Read the model definition and answer for the solid it produces. Units are mm, in the model's axes. Face numbers are marked on the shaded views. Coordinates: 2 decimals unless noted, no trailing zeros. Loops run counter-clockwise (first coordinate to the right, second up) from the corner with the lowest first, then second, coordinate; pieces in that order, holes last.
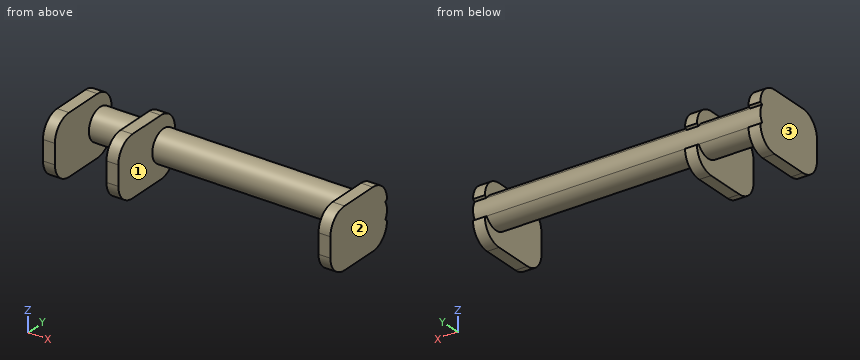
from build123d import *

# Parameters (mm, degrees)
SCHIZZO1_R                   = 8
ESTRUSIONE_ESTRUSIONE1_DEPTH = 145
ESTRUSIONE_ESTRUSIONE2_DEPTH = 6
RIPETIZIONE_A_L1_COUNT       = 2
RIPETIZIONE_A_L1_PITCH       = 32
RIPETIZIONE_A_L2_COUNT       = 2
RIPETIZIONE_A_L2_PITCH       = 139
EXTRUDE2_DEPTH               = 150.244765402


with BuildPart() as part:
    # Schizzo1 → Estrusione-Estrusione1 (new body)
    with BuildSketch(Plane(origin=(0, 0, 0), x_dir=(0, 0, -1), z_dir=(1, 0, 0))):
        Circle(SCHIZZO1_R)
    extrude(amount=ESTRUSIONE_ESTRUSIONE1_DEPTH)

    # Schizzo2 → Estrusione-Estrusione2 (add)
    with BuildSketch(Plane.ZY):
        with BuildLine():
            Line((-5, 8), (5, 8))
            ThreePointArc((5, 8), (12.071067812, 5.071067812), (15, -2))
            Line((15, -2), (15, -22))
            ThreePointArc((15, -22), (12.071067812, -29.071067812), (5, -32))
            Line((5, -32), (-5, -32))
            ThreePointArc((-5, -32), (-12.071067812, -29.071067812), (-15, -22))
            Line((-15, -22), (-15, -2))
            ThreePointArc((-15, -2), (-12.071067812, 5.071067812), (-5, 8))
        make_face()
    estrusione_estrusione2 = extrude(amount=-ESTRUSIONE_ESTRUSIONE2_DEPTH)

    # Ripetizione a L1: Estrusione-Estrusione2 ×2
    with Locations(*[(i * RIPETIZIONE_A_L1_PITCH, 0, 0) for i in range(1, RIPETIZIONE_A_L1_COUNT)]):
        add(estrusione_estrusione2)

    # Ripetizione a L2: Estrusione-Estrusione2 ×2
    with Locations(*[(i * RIPETIZIONE_A_L2_PITCH, 0, 0) for i in range(1, RIPETIZIONE_A_L2_COUNT)]):
        add(estrusione_estrusione2)

    # Sketch1 → Extrude2 (cut, through all)
    with BuildSketch(Plane.ZY):
        with BuildLine():
            Line((-5, 8), (-4.23999152, 6.783986432))
            ThreePointArc((-4.23999152, 6.783986432), (0, 8), (4.23999152, 6.783986432))
            Line((4.23999152, 6.783986432), (5, 8))
            Line((5, 8), (5, 8.502646834))
            Line((5, 8.502646834), (-5, 8.502646834))
            Line((-5, 8.502646834), (-5, 8))
        make_face()
    extrude(amount=-EXTRUDE2_DEPTH, mode=Mode.SUBTRACT)


solid = part.part
Item 1: A cutting plane is placed at C-C on z = 0. Determine the outline of the cut face in (x, y), then the cut area to 3 significant figures.
Numbers:
outline: (0, -32) - (6, -32) - (6, -8) - (32, -8) - (32, -32) - (38, -32) - (38, -8) - (139, -8) - (139, -32) - (145, -32) - (145, 8) - (0, 8) - close
area: 2,750 mm2
Item 2: A cutting plane is placed at B-B on y = -11.5. Determine the outline of the cut face in (x, z), then the cut area to 3 significant figures.
Numbers:
outline: (0, -15) - (6, -15) - (6, 15) - (0, 15) - close; (32, -15) - (38, -15) - (38, 15) - (32, 15) - close; (139, -15) - (145, -15) - (145, 15) - (139, 15) - close
area: 540 mm2
Item 3: Determine the mould class of the marked faces 1, 2 and 3 for opening direction X: released by +X, released by -X, zero draft, split by the parting line, or undercut.
Numbers:
face 1: undercut
face 2: released by +X
face 3: released by -X
Item 4: Given pin 1 (12 mm diameter, centred on x = 20, z = -2, fed in from -Y); pin 2 (12 mm diameter, centred on x = 17.5, y = -4.5, fed in from -Z); pin 3 (9 mm diameter, centred on y = -14, z = -3.5, fed in from -X); pin 4 (4 mm diameter, centred on x = 103.5, z = 6, fed in from +Y), each flat-ended and moving along its own axis, determine where each tip first touches the part or whether it passes through.
Numbers:
pin 1: stops at y = -8
pin 2: stops at z = -8
pin 3: stops at x = 0
pin 4: stops at y = 6.93
Item 5: A cutting plane is placed at D-D on x = 43. Determine the outline of the cut face in (y, z), then the cut area to 3 significant figures.
Numbers:
outline: circle Ø16 at (0, 0)
area: 201 mm2
Item 6: Find the intervals of material crossed by line 1 along X through (y, z) = (-19, 1.5); line 2 along Y through (x, z) = (109, 0.5); line 3 along Z through (x, y) = (55, -7), in increasing order.
Numbers:
line 1: x = 0 to 6, 32 to 38, 139 to 145
line 2: y = -7.98 to 7.98
line 3: z = -3.87 to 3.87
Item 7: A cutting plane is placed at A-A on z = -11. Determine the outline of the cut face in (x, y).
Numbers:
outline: (0, -30) - (6, -30) - (6, 6) - (0, 6) - close; (32, -30) - (38, -30) - (38, 6) - (32, 6) - close; (139, -30) - (145, -30) - (145, 6) - (139, 6) - close
